```python
from build123d import *

# Parameters (mm, degrees)
SKETCH_1_R       = 188.695873506
SKETCH_1_R_2     = 170
EXTRUDE_4_DEPTH  = 15
SKETCH_1_8_R     = 203.2
SKETCH_1_8_R_2   = 188.695873506
EXTRUDE_5_DEPTH  = 18
CHAMFER_1_SIZE   = 15
CHAMFER_1_SIZE_2 = 4.019237886
FILLET_1_R       = 18
FILLET_2_R       = 1.75


# Some blends are built 0.0001 mm under size
with BuildPart() as part:
    # ｽｹｯﾁ1 → ﾎﾞｽ - 押し出し4 (new body)
    with BuildSketch(Plane(origin=(0, 0, 0), x_dir=(1, 0, 0), z_dir=(0, 1, 0))):
        with Locations(Location((0, 0, 0), (0, 0, 270))):
            Circle(SKETCH_1_R)
        with Locations(Location((0, 0, 0), (0, 0, 270))):
            Circle(SKETCH_1_R_2, mode=Mode.SUBTRACT)
    extrude_4 = extrude(amount=EXTRUDE_4_DEPTH)

    # ｽｹｯﾁ1<8> → ﾎﾞｽ - 押し出し5 (add)
    with BuildSketch(Plane(origin=(0, 0, 0), x_dir=(1, 0, 0), z_dir=(0, 1, 0))):
        with Locations(Location((0, 0, 0), (0, 0, 270))):
            Circle(SKETCH_1_8_R)
        with Locations(Location((0, 0, 0), (0, 0, 270))):
            Circle(SKETCH_1_8_R_2, mode=Mode.SUBTRACT)
    extrude_5 = extrude(amount=EXTRUDE_5_DEPTH)

    # ﾐﾗｰ1: ﾎﾞｽ - 押し出し4, ﾎﾞｽ - 押し出し5 across plane
    add(extrude_4.mirror(Plane.ZX))
    add(extrude_5.mirror(Plane.ZX))

    # 面取り1
    # the kernel refuses this chamfer: 15, 4.019237886 mm, written as the material it adds along each edge
    with BuildSketch(Plane(origin=(0, -15, 0), x_dir=(0, 0, 1), z_dir=(-1, 0, 0))) as chamfer_1_piece_1_section:
        Polygon((188.695873506 - CHAMFER_1_SIZE, 0), (188.695873506, -CHAMFER_1_SIZE_2), (188.695873506, 0), align=None)
    chamfer_1_piece_1 = revolve(axis=Axis((0, -15, 0), (0, 1, 0)), mode=Mode.PRIVATE)
    chamfer_1_piece_1 = split(chamfer_1_piece_1, bisect_by=Plane(origin=(0, -18, -179.092170597), z_dir=(0, 1, 0)), keep=Keep.TOP, mode=Mode.PRIVATE)
    add(chamfer_1_piece_1)
    with BuildSketch(Plane(origin=(0, 15, 0), x_dir=(0, 0, 1), z_dir=(-1, 0, 0))) as chamfer_1_piece_2_section:
        Polygon((188.695873506 - CHAMFER_1_SIZE, 0), (188.695873506, CHAMFER_1_SIZE_2), (188.695873506, 0), align=None)
    chamfer_1_piece_2 = revolve(axis=Axis((0, 15, 0), (0, 1, 0)), mode=Mode.PRIVATE)
    chamfer_1_piece_2 = split(chamfer_1_piece_2, bisect_by=Plane(origin=(0, 18, -179.092170597), z_dir=(0, -1, 0)), keep=Keep.TOP, mode=Mode.PRIVATE)
    add(chamfer_1_piece_2)

    # ﾌｨﾚｯﾄ1
    fillet_1_edges = [part.edges().sort_by_distance(p)[0] for p in [
        (0, -18, -203.2),
        (0, 18, -203.2),
    ]]
    fillet(fillet_1_edges, radius=FILLET_1_R - 0.0001)  # a hair under: the kernel refuses the full size

    # ﾌｨﾚｯﾄ2
    fillet_2_edges = [part.edges().sort_by_distance(p)[0] for p in [
        (0, -15, -170),
        (0, 15, -170),
    ]]
    fillet(fillet_2_edges, radius=FILLET_2_R)


solid = part.part
```
For this review, take the finished solid that the model builds, in its own axes (mm). A direction names the side the tool comes from. Round coordinates to 2 decimals unless told otherwise and drop trailing zeros. Write each loop counter-clockwise with the first axis right and the second up, starting at its lowest first coordinate (ties: lowest second). Pieces come first, ordered by that corner, then holes. Notation, with made-up numbers: M 23.25,43.5 L 76.25,43.5 A36 ccw 76.25,80.5 Z; hole C -27.75,1 d5. An arc over 180 degrees is marked long. One line per item, written item: value. Start each with the question number.
(1) We need section C-C (y = 8). Give the boundary of the cut face in (x, z), and give its area (3 significant figures).
(2) Machinability: for faces 1 (the cylindrical face through (-103.44, -0.19, -134.91)), 2 (the flat face through (39, 15, -168)), 3 (the flat face through (39, -15, -168)), which of the approach directions +Z, -Z, +X, -X, +Y, -Y give a long, thin tool a straight path to every point of the face, cutting with its end or side? Answer none if there is none.
(3) Wall thickness on line 1 (X direction, y = -1, z = 0); line 2 (X direction, y = 0, z = 0); line 3 (Z direction, x = 21, y = 9.5): over which ranges is each line inside the solid? List them lowest first.
(4) Insertion check: pin 1 (8 mm diameter, centred on y = -12, z = 86.5, fed in from +X); pin 2 (2 mm diameter, centred on x = 133.5, y = 1.5, fed in from -Z); pin 3 (1.5 mm diameter, centred on x = 118.5, y = 0, fed in from +Z). Each pin has a flat end and moves straight along its axis. Give the tip position at first contact, or say it passes through.
Result:
1. outline: C 0,0 d402.65; hole C 0,0 d340
1. area: 36,500 mm²
2. face 1: +Y, -Y
2. face 2: +Y
2. face 3: -Y
3. line 1: -203.17 to -170, 170 to 203.17
3. line 2: -203.2 to -170, 170 to 203.2
3. line 3: -199.39 to -168.7, 168.7 to 199.39
4. pin 1: x = 182.45
4. pin 2: z = -153.98
4. pin 3: z = 165.61
